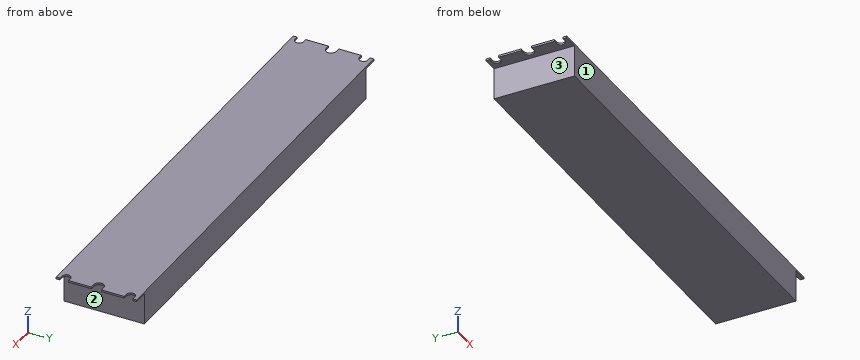
```python
from build123d import *

# Parameters (mm, degrees)
SKETCH1_W           = 423.926
SKETCH1_H           = 31.75
BOSS_EXTRUDE1_DEPTH = 76.2
SKETCH5_W           = 13.97
SKETCH5_H           = 76.2
CUT_EXTRUDE5_DEPTH  = 29.972
SKETCH6_R           = 4.064
SKETCH6_R_2         = 4.826
CUT_EXTRUDE6_DEPTH  = 416.56
CUT_EXTRUDE7_DEPTH  = 2.778


with BuildPart() as part:
    # Sketch1 → Boss-Extrude1 (new body)
    with BuildSketch(Plane(origin=(0, 0, 0), x_dir=(1, 0, 0), z_dir=(0, 1, 0))):
        with Locations((211.963, 15.875)):
            Rectangle(SKETCH1_W, SKETCH1_H)
    extrude(amount=BOSS_EXTRUDE1_DEPTH)

    # Sketch5 → Cut-Extrude5 (cut)
    with BuildSketch(Plane(origin=(0, 0, -31.75), x_dir=(-1, 0, 0), z_dir=(0, 0, -1))):
        with Locations((-416.941, 38.1)):
            Rectangle(SKETCH5_W, SKETCH5_H)
        with Locations((-6.985, 38.1)):
            Rectangle(SKETCH5_W, SKETCH5_H)
    extrude(amount=-CUT_EXTRUDE5_DEPTH, mode=Mode.SUBTRACT)

    # Sketch6 → Cut-Extrude6 (cut)
    with BuildSketch(Plane(origin=(0, 0, -1.778), x_dir=(-1, 0, 0), z_dir=(0, 0, -1))):
        with Locations((-3.81, 7.62)):
            Circle(SKETCH6_R)
        with Locations((-3.81, 68.58)):
            Circle(SKETCH6_R)
        with Locations((-4.445, 38.1)):
            Circle(SKETCH6_R_2)
        with Locations((-420.37, 7.62)):
            Circle(SKETCH6_R)
        with Locations((-420.116, 68.58)):
            Circle(SKETCH6_R)
        with Locations((-419.481, 38.1)):
            Circle(SKETCH6_R_2)
    extrude(amount=-CUT_EXTRUDE6_DEPTH, mode=Mode.SUBTRACT)

    # Sketch8 → Cut-Extrude7 (cut, through all)
    with BuildSketch(Plane(origin=(0, 0, -1.778), x_dir=(-1, 0, 0), z_dir=(0, 0, -1))):
        Polygon((-419.862, 72.636054733), (-423.926, 72.636054733), (-423.926, 69.994212148), align=None)
        Polygon((-419.862, 64.523945267), (-423.926, 64.269447715), (-423.926, 67.165787852), align=None)
        Polygon((-419.481, 42.926), (-423.926, 42.926), (-423.926, 39.979428371), align=None)
        Polygon((-419.481, 33.274), (-423.926, 33.274), (-423.926, 36.220571629), align=None)
        Polygon((-420.37, 11.684), (-423.926, 11.684), (-423.926, 9.58747554), align=None)
        Polygon((-420.37, 3.556), (-423.926, 3.556), (-423.926, 5.65252446), align=None)
        Polygon((-3.81, 72.644), (0, 72.644), (0, 69.994212148), align=None)
        Polygon((-3.81, 64.516), (0, 64.516), (0, 67.165787852), align=None)
        Polygon((-4.445, 42.926), (0, 42.926), (0, 39.979428371), align=None)
        Polygon((-4.445, 33.274), (0, 33.274), (0, 36.220571629), align=None)
        Polygon((-3.81, 11.684), (0, 11.684), (0, 9.034212148), align=None)
        Polygon((-3.81, 3.556), (0, 3.556), (0, 6.205787852), align=None)
    extrude(amount=-CUT_EXTRUDE7_DEPTH, mode=Mode.SUBTRACT)


solid = part.part
```
Could you check a few things on this model? Use its own coordinates, in mm. Face numbers are marked on the shaded views. A direction names the side the tool comes from. Coordinates: 2 decimals unless noted, no trailing zeros. Loops run counter-clockwise (first coordinate to the right, second up) from the corner with the lowest first, then second, coordinate; pieces in that order, holes last.
1) Imagine slicing it at B-B (y = 68.58). List the corners of the cut face in (x, z) for me, and give its area (3 significant figures).
Reported:
outline: (7.87, -1.78) - (13.97, -1.78) - (13.97, -31.75) - (409.96, -31.75) - (409.96, -1.78) - (416.05, -1.78) - (416.05, 0) - (7.87, 0) - close
area: 12,600 mm2
2) Please list where this line runs through material, in increasing order: line 1 along X through (y, z) = (38, -28).
Reported:
line 1: x = 13.97 to 409.96
3) Will these pins go through, and if not, where does the flat tip stop? pin 1 Ø3 at (y, z) = (62, -24.5) entering from -X; pin 2 Ø7 at (x, y) = (419.5, 41.5) entering from -Z.
Reported:
pin 1: stops at x = 13.97
pin 2: stops at z = -1.78
4) Imagine slicing it at C-C (z = -25). List the corners of the cut face in (x, y) for me, and give its area (3 significant figures).
Reported:
outline: (13.97, 0) - (409.96, 0) - (409.96, 76.2) - (13.97, 76.2) - close
area: 30,200 mm2
5) Imagine slicing it at A-A (y = 24). List the corners of the cut face in (x, z) for me, and give its area (3 significant figures).
Reported:
outline: (0, -1.78) - (13.97, -1.78) - (13.97, -31.75) - (409.96, -31.75) - (409.96, -1.78) - (423.93, -1.78) - (423.93, 0) - (0, 0) - close
area: 12,600 mm2
6) Which directions (+Z, -Z, +X, -X, +Y, -Y) give clear straight access to the entire face, cutting with the end or side of a thin tool? Please do the marked faces 1, 2 and 3.
Reported:
face 1: +Z, -Z, +X, -X, -Y
face 2: -Z, +X, +Y, -Y
face 3: -Z, -X, +Y, -Y
